Can you work these out from the model? Positions are in its coordinate system, mm. A direction names the side the tool comes from. Give positions to 0.01 mm unless a question says otherwise; leave off trailing zeros. Order: outer loops, then holes, each group sorted by start corner. A loop starts at its lowest first (then second) coordinate and runs counter-clockwise, first axis right, second up. Notation, with made-up numbers: M -31,78 L 24,78 A6 ccw 24,83 Z; hole C 41,-1.75 d7. An arc over 180 degrees is marked long. Answer as a JSON object with one key per item and string values.
```python
from build123d import *

# Parameters (mm, degrees)
SKETCH1_W           = 47
SKETCH1_H           = 47
BOSS_EXTRUDE1_DEPTH = 2
BOSS_EXTRUDE2_DEPTH = 5


with BuildPart() as part:
    # Sketch1 → Boss-Extrude1 (new body)
    with BuildSketch(Plane.XY):
        with Locations((23.5, 23.5)):
            Rectangle(SKETCH1_W, SKETCH1_H)
    extrude(amount=BOSS_EXTRUDE1_DEPTH)

    # Sketch2 → Boss-Extrude2 (add)
    with BuildSketch(Plane.XY.offset(2)):
        Polygon((5, 47), (5, 45), (2, 45), (2, 42), (0, 42), (0, 47), align=None)
        Polygon((42, 47), (42, 45), (45, 45), (45, 42), (47, 42), (47, 47), align=None)
        Polygon((0, 5), (0, 0), (5, 0), (5, 2), (2, 2), (2, 5), align=None)
        Polygon((47, 5), (45, 5), (45, 2), (42, 2), (42, 0), (47, 0), align=None)
    extrude(amount=BOSS_EXTRUDE2_DEPTH)


solid = part.part
```
1) Thinking about a two-plate mould opening in Y: for faces 4 (the face through (44, 2, 4)), 5 (the face through (23, 0, 1)), 6 (the face through (5, 1, 4)), which applies, pulls with the +Y half, pulls with the -Y half, needs draft (parallel to the pull), parting line crosses it, or undercut?
Results found:
{"face 4": "undercut", "face 5": "pulls with the -Y half", "face 6": "needs draft"}
2) I want a section at B-B on y = 36. Write out the boundary of the cut face in (x, z).
Results found:
{"outline": "M 0,0 L 47,0 L 47,2 L 0,2 Z"}
3) I'm going to push a flat-ended pin straight in: pin 1 Ø23.5 at (x, y) = (19, 32) entering from +Z. Where does the tip first touch, or does it pass through?
Results found:
{"pin 1": "stops at z = 2"}
4) I want a section at A-A on z = 4. Write out the boundary of the cut face in (x, y).
Results found:
{"outline": "M 0,0 L 5,0 L 5,2 L 2,2 L 2,5 L 0,5 Z; M 0,42 L 2,42 L 2,45 L 5,45 L 5,47 L 0,47 Z; M 42,0 L 47,0 L 47,5 L 45,5 L 45,2 L 42,2 Z; M 42,45 L 45,45 L 45,42 L 47,42 L 47,47 L 42,47 Z"}
5) I need wall thicknesses on L1, parallel to X at y = 45.5, z = 4; L2, parallel to X at y = 2.5, z = 4.75; L3, parallel to Z at x = 37.5, y = 44. Which ranges of each line are inside material? Lowest first, please.
Results found:
{"L1": "x = 0 to 5, 42 to 47", "L2": "x = 0 to 2, 45 to 47", "L3": "z = 0 to 2"}
6) For faces 1 (the face through (46, 42, 4)), 2 (the face through (45, 4, 4)), 3 (the face through (42, 1, 4)), which set-ups out of +Z, -Z, +X, -X, +Y, -Y let a thin tool reach every point of the face, with its end or its side?
Results found:
{"face 1": "+Z, +X, -X", "face 2": "+Z", "face 3": "+Z, +Y, -Y"}
